Could you check a few things on this model? Use its own coordinates, in mm. A direction names the side the tool comes from. Round coordinates to 2 decimals unless told otherwise and drop trailing zeros. Order: outer loops, then holes, each group sorted by start corner. A loop starts at its lowest first (then second) coordinate and runs counter-clockwise, first axis right, second up. Notation, with made-up numbers: (56.5, 73) -> (106.5, 73) arc R17 ccw to (106.5, 99) -> close; hole circle Ø8 at (52.25, 53.5). An arc over 180 degrees is marked (long way). One line per question, with ' | ' between items.
```python
from build123d import *

# Parameters (mm, degrees)
SKETCH_1_R          = 41
SKETCH_1_R_2        = 1.525
EXTRUDE_1_DEPTH     = 2
EXTRUDE_3_DEPTH     = 2
FILLET_1_R          = 2
EXTRUDE_5_DEPTH     = 2
CUT_EXTRUDE_1_DEPTH = 10
FILLET_3_R          = 2


with BuildPart() as part:
    # 草图1 → 凸台-拉伸1 (new body)
    with BuildSketch(Plane(origin=(0, 0, 0), x_dir=(1, 0, 0), z_dir=(0, 1, 0))):
        with BuildLine():
            Line((-54, 0), (-54, 54))
            Line((-54, 54), (-10, 54))
            Line((-10, 54), (-10, 53.065996646))
            ThreePointArc((-10, 53.065996646), (41.569219382, -34.467375879), (-54, 0))
        make_face()
        with Locations(Location((0, 0, 0), (0, 0, 270))):
            Circle(SKETCH_1_R, mode=Mode.SUBTRACT)
        with Locations(Location((-15, 46.647615159, 0), (0, 0, 270))):
            Circle(SKETCH_1_R_2, mode=Mode.SUBTRACT)
        with Locations(Location((0, 49, 0), (0, 0, 270))):
            Circle(SKETCH_1_R_2, mode=Mode.SUBTRACT)
        with Locations(Location((49, 0, 0), (0, 0, 270))):
            Circle(SKETCH_1_R_2, mode=Mode.SUBTRACT)
        with Locations(Location((0, -49, 0), (0, 0, 270))):
            Circle(SKETCH_1_R_2, mode=Mode.SUBTRACT)
        with Locations(Location((-49, 0, 0), (0, 0, 270))):
            Circle(SKETCH_1_R_2, mode=Mode.SUBTRACT)
        with Locations(Location((-49, 46.647615159, 0), (0, 0, 270))):
            Circle(SKETCH_1_R_2, mode=Mode.SUBTRACT)
    extrude(amount=EXTRUDE_1_DEPTH)

    # 草图2 → 凸台-拉伸3 (add)
    with BuildSketch(Plane(origin=(0, 0, 0), x_dir=(1, 0, 0), z_dir=(0, 1, 0))):
        with BuildLine():
            Line((-41, 0), (-37.46998799, 0))
            ThreePointArc((-37.46998799, 0), (-36.430757506, 0.418334617), (-35.971188471, 1.44))
            ThreePointArc((-35.971188471, 1.44), (-25.240038288, 25.669835746), (-0.832477451, 35.990373453))
            ThreePointArc((-0.832477451, 35.990373453), (-0.105240976, 36.197891356), (0.428319211, 36.733848535))
            Line((0.428319211, 36.733848535), (2.860015424, 40.900126061))
            ThreePointArc((2.860015424, 40.900126061), (-27.961932763, 29.985501766), (-41, 0))
        make_face()
    extrude(amount=EXTRUDE_3_DEPTH)

    # 圆角1
    fillet_1_edges = [part.edges().sort_by_distance(p)[0] for p in [
        (2.860015424, 1, -40.900126061),
        (-41, 1, 0),
    ]]
    fillet(fillet_1_edges, radius=FILLET_1_R)

    # 草图4 → 凸台-拉伸5 (add)
    with BuildSketch(Plane.XZ):
        with BuildLine():
            Line((-38.948684188, 0), (-37.46998799, 0))
            ThreePointArc((-37.46998799, 0), (-36.430757506, -0.418334617), (-35.971188471, -1.44))
            ThreePointArc((-35.971188471, -1.44), (-34.952758609, 8.620015408), (-31.176914536, 18))
            Line((-31.176914536, 18), (-35.507041555, 20.5))
            ThreePointArc((-35.507041555, 20.5), (-39.317748075, 11.623884304), (-40.946052608, 2.102564103))
            ThreePointArc((-40.946052608, 2.102564103), (-40.398706292, 0.622525537), (-38.948684188, 0))
        make_face()
    extrude(amount=-EXTRUDE_5_DEPTH)

    # 草图5 → 切除-拉伸1 (cut)
    with BuildSketch(Plane.XZ):
        with BuildLine():
            Line((-16.167566472, 51.522905531), (-5.300581056, 40.655920116))
            ThreePointArc((-5.300581056, 40.655920116), (-28.991378029, 28.991378029), (-40.655920116, 5.300581056))
            Line((-40.655920116, 5.300581056), (-51.522905531, 16.167566472))
            ThreePointArc((-51.522905531, 16.167566472), (-38.183766184, 38.183766184), (-16.167566472, 51.522905531))
        make_face()
    extrude(amount=-CUT_EXTRUDE_1_DEPTH, mode=Mode.SUBTRACT)

    # 圆角3
    fillet_3_edges = [part.edges().sort_by_distance(p)[0] for p in [
        (-5.300581056, 1, 40.655920116),
        (-40.655920116, 1, 5.300581056),
        (-35.507041555, 1, 20.5),
        (-31.176914536, 1, 18),
        (-51.522905531, 1, 16.167566472),
        (-16.167566472, 1, 51.522905531),
    ]]
    fillet(fillet_3_edges, radius=FILLET_3_R)


solid = part.part
```
1. I want a section at A-A on x = 49. List the corners of the cut face in (y, z) for me (3 decimals).
From the geometry:
outline: (0, -22.694) -> (2, -22.694) -> (2, -1.525) -> (0, -1.525) -> close; (0, 1.525) -> (2, 1.525) -> (2, 22.694) -> (0, 22.694) -> close
2. I want a section at C-C on y = 0.9. List the corners of the cut face in (x, z) for me (3 decimals).
From the geometry:
outline: (-54, -54) -> (-10, -54) -> (-10, -53.066) arc R54 ccw (long way) to (-12.807, 52.459) arc R2 ccw to (-13.747, 49.102) -> (-5.987, 41.342) arc R2 ccw to (-4.36, 40.768) arc R41 cw to (4.152, -40.789) arc R2 cw to (2.222, -39.808) -> (0.428, -36.734) arc R1.5 ccw to (-0.832, -35.99) arc R36 cw to (-32.081, 16.334) arc R2 ccw to (-32.863, 18.974) -> (-33.731, 19.474) arc R2 ccw to (-36.512, 18.652) arc R41 ccw to (-40.003, 8.989) arc R2 cw to (-43.368, 8.013) -> (-49.102, 13.747) arc R2 ccw to (-52.459, 12.807) arc R54 ccw to (-54, 0) -> close; hole circle Ø3.05 at (-49, -46.648); hole circle Ø3.05 at (-49, 0); hole circle Ø3.05 at (-15, -46.648); hole circle Ø3.05 at (0, -49); hole circle Ø3.05 at (0, 49); hole circle Ø3.05 at (49, 0)
3. I want a section at B-B on z = -14.5. List the corners of the cut face in (x, y) for me.
From the geometry:
outline: (-54, 0) -> (-32.95, 0) -> (-32.95, 2) -> (-54, 2) -> close; (38.35, 0) -> (52.02, 0) -> (52.02, 2) -> (38.35, 2) -> close
4. On a 3-axis mill with a long thin cutter (end or side, diameter ignored), from which of +Z, -Z, +X, -X, +Y, -Y can I reach the whole of each face in a straight line? I mean faces 1 (the face through (-46.195, 0.986, 10.84)), 2 (the face through (-13, 2, -35)), 3 (the face through (40.675, 0.986, 5.153)). Say none if no direction works.
From the geometry:
face 1: +Z, +Y, -Y | face 2: +Z, -Z, +X, -X, +Y | face 3: +Y, -Y
5. I want a section at D-D on x = -21.5. List the corners of the cut face in (y, z) for me.
From the geometry:
outline: (0, -54) -> (2, -54) -> (2, -28.87) -> (0, -28.87) -> close
6. If we mould it in two halves opening along Z, with no side actions, what happens to faces 4 (the face through (-9.921, 0.986, 45.276)), 5 (the face through (54, 1, 0)), 6 (the face through (-38.536, 0.986, 13.998))? For each: pulls with the +Z half, pulls with the -Z half, needs draft (parallel to the pull), parting line crosses it, or undercut.
From the geometry:
face 4: undercut | face 5: parting line crosses it | face 6: pulls with the +Z half
7. I'm going to push flat-ended pins straight in: pin 1 (2.5 mm diameter, centred on x = 0, z = 49, fed in from -Y); pin 2 (1 mm diameter, centred on y = 1, z = 20.5, fed in from +X); pin 3 (1 mm diameter, centred on y = 1, z = 18, fed in from -X). Where does each tip first touch, or does it pass through?
From the geometry:
pin 1: passes through | pin 2: stops at x = 50.16 | pin 3: stops at x = -37.08
8. I need wall thicknesses on probe 1 along X at (y, z) = (0.5, 11.5); probe 2 along Z at (x, y) = (33, 1); probe 3 along Z at (x, y) = (-11, 1.75). Which ranges of each line are inside material? Lowest first, please.
From the geometry:
probe 1: x = -52.76 to -46.86, -39.35 to -34.11, 39.35 to 52.76 | probe 2: z = -42.74 to -24.33, 24.33 to 42.74 | probe 3: z = -54 to -34.28, 46.36 to 52.87
